```python
from build123d import *

# Parameters (mm, degrees)
BASE_FLANGE1_DEPTH    = 2
EDGE_FLANGE1_DEPTH    = 12
M5_CLEARANCE_HOLE1_D  = 5.8
M3_CLEARANCE_HOLE1_D  = 3.6
SKETCH14_R            = 1.25
CUT_EXTRUDE1_DEPTH    = 41.360872141
BREAK_CORNER1_START   = -8
BREAK_CORNER1_DEPTH   = 2
BREAK_CORNER1_2_DEPTH = 2


# Read off the part's stored shape, not the designer's step: Break-Corner1
# Sheet-metal steps are written as plain solids
with BuildPart() as part:
    # Sketch1 → Base-Flange1 (new body)
    with BuildSketch(Plane(origin=(0, 0, 0), x_dir=(1, 0, 0), z_dir=(0, 1, 0))):
        with BuildLine():
            Line((0, 0), (0, 12))
            Line((0, 12), (-34, 12))
            Line((-34, 12), (-34, 0))
            Line((-34, 0), (-13, -13))
            Line((-13, -13), (-10, -13))
            Line((-10, -13), (-10, -1))
            ThreePointArc((-10, -1), (-10.5, -0.5), (-10, 0))
            Line((-10, 0), (0, 0))
        make_face()
    extrude(amount=BASE_FLANGE1_DEPTH)

    # Edge-Flange1 section (across the edge) → Edge-Flange1 (add)
    with BuildSketch(Plane(origin=(-8, 0, 1), x_dir=(-1, 0, 0), z_dir=(0, 0, 1))):
        with BuildLine():
            Line((-2, 2), (-2, 26))
            Line((-2, 26), (0, 26))
            Line((0, 26), (0, 2))
            ThreePointArc((0, 2), (0.585786438, 0.585786438), (2, 0))
            Line((2, 0), (2, -2))
            ThreePointArc((2, -2), (-0.828427125, -0.828427125), (-2, 2))
        make_face()
    extrude(amount=EDGE_FLANGE1_DEPTH)

    # M5 Clearance Hole1 (through all)
    with Locations(Plane(origin=(0, 2, 0), x_dir=(1, 0, 0), z_dir=(0, 1, 0))):
        with Locations((-29, 6), (-5, 6)):
            Hole(M5_CLEARANCE_HOLE1_D / 2)

    # M3 Clearance Hole1 (through all)
    with Locations(Plane(origin=(-6, 0, 0), x_dir=(0, 0, -1), z_dir=(1, 0, 0))):
        with Locations((-7, -21)):
            Hole(M3_CLEARANCE_HOLE1_D / 2)

    # Sketch14 → Cut-Extrude1 (cut, through all)
    with BuildSketch(Plane(origin=(-6, 0, 0), x_dir=(0, 0, -1), z_dir=(1, 0, 0))):
        with Locations(Location((-7, -5, 0), (0, 0, 90))):
            Circle(SKETCH14_R)
    extrude(amount=-CUT_EXTRUDE1_DEPTH, mode=Mode.SUBTRACT)

    # Break-Corner1 outline → Break-Corner1 (cut)
    with BuildSketch(Plane.YZ.offset(BREAK_CORNER1_START)):
        with BuildLine():
            Line((-26, 1), (-24, 1))
            ThreePointArc((-24, 1), (-25.414213562, 1.585786438), (-26, 3))
            Line((-26, 3), (-26, 1))
        make_face()
        with BuildLine():
            Line((-26, 13), (-26, 11))
            ThreePointArc((-26, 11), (-25.414213562, 12.414213562), (-24, 13))
            Line((-24, 13), (-26, 13))
        make_face()
    extrude(amount=BREAK_CORNER1_DEPTH, mode=Mode.SUBTRACT)

    # Break-Corner1 2 outline → Break-Corner1 2 (cut)
    with BuildSketch(Plane(origin=(0, 0, 0), x_dir=(1, 0, 0), z_dir=(0, 1, 0))):
        with BuildLine():
            Line((-13, -13), (-12.431049528, -13))
            ThreePointArc((-12.431049528, -13), (-12.978287782, -12.923676244), (-13.483758757, -12.700530293))
            Line((-13.483758757, -12.700530293), (-13, -13))
        make_face()
        with BuildLine():
            Line((0, 0), (0, 2))
            ThreePointArc((0, 2), (-0.585786438, 0.585786438), (-2, 0))
            Line((-2, 0), (0, 0))
        make_face()
        with BuildLine():
            Line((0, 12), (-2, 12))
            ThreePointArc((-2, 12), (-0.585786438, 11.414213562), (0, 10))
            Line((0, 10), (0, 12))
        make_face()
        with BuildLine():
            Line((-34, 12), (-34, 10))
            ThreePointArc((-34, 10), (-33.414213562, 11.414213562), (-32, 12))
            Line((-32, 12), (-34, 12))
        make_face()
        with BuildLine():
            Line((-34, 0), (-33.052709229, -0.586418096))
            ThreePointArc((-33.052709229, -0.586418096), (-33.747200398, 0.14082356), (-34, 1.114112197))
            Line((-34, 1.114112197), (-34, 0))
        make_face()
    extrude(amount=BREAK_CORNER1_2_DEPTH, mode=Mode.SUBTRACT)


solid = part.part
```
The listing builds one solid part. Answer for the finished solid, in the listing's coordinates (mm). A direction names the side the tool comes from. Give positions to 0.01 mm unless a question says otherwise; leave off trailing zeros. Write each loop counter-clockwise with the first axis right and the second up, starting at its lowest first coordinate (ties: lowest second). Pieces come first, ordered by that corner, then holes. Notation, with made-up numbers: (1.5, -24) - (35.5, -24) arc R35 ccw to (35.5, 13) - close; hole circle Ø2 at (-27, 43). An arc over 180 degrees is marked (long way). Use one line per item in the form item = value. Start each with the question number.
1) Find section B-B on x = -5. Determine the outline of the cut face in (y, z), plus the area to 3 significant figures.
2) Find section C-C on y = -5. Determine the outline of the cut face in (x, z).
3) The mould has two halves that part along Z. Classify faces 1 (the face through (-17, 1, -12)), 2 (the face through (-12.971, 0.986, 12.926)), 3 (the face through (-10.5, 1, 0.5)): pulls with the +Z half, pulls with the -Z half, needs draft (parallel to the pull), parting line crosses it, or undercut.
4) Find section A-A on z = -6. Determine the outline of the cut face in (x, y).
5) Find section D-D on z = 10.25. Determine the outline of the cut face in (x, y), plus the area to 3 significant figures.
6) Consider line 1 along Z through (x, y) = (-7, -5); line 2 along Z through (x, y) = (-5, 0.8); line 3 along X through (y, z) = (0.75, -8.25). Determine where each line is inside the solid, lowest interval first. Write a range as from..to.
7) Flat-ended cylindrical pins translate along their axes: pin 1 Ø2 at (x, z) = (-25, -5.5) entering from -Y; pin 2 Ø9.5 at (y, z) = (-10.5, 8) entering from +X; pin 3 Ø4.5 at (x, y) = (-8, -10) entering from -Z. Find the tip coordinate at first contact, or state that the pin passes through.
8) A tool of negligible diameter and unlimited length cuts with its end or side. For faces 4 (the face through (-6, 1, 0)), 5 (the face through (-8, -14, 7)), 6 (the face through (-7.203, 0.859, 6.916)), from which of +Z, -Z, +X, -X, +Y, -Y can it reach the whole face along a straight path? Write none if from no direction.
Geometry results:
q1.outline = (0, -12) - (2, -12) - (2, -8.9) - (0, -8.9) - close; (0, -3.1) - (2, -3.1) - (2, 0) - (0, 0) - close
q1.area = 12.4 mm2
q2.outline = (-8, 1) - (-6, 1) - (-6, 5.75) - (-8, 5.75) - close; (-8, 8.25) - (-6, 8.25) - (-6, 13) - (-8, 13) - close
q3.face_1 = pulls with the -Z half
q3.face_2 = pulls with the +Z half
q3.face_3 = undercut
q4.outline = (-34, 0) - (-31.9, 0) - (-31.9, 2) - (-34, 2) - close; (-26.1, 0) - (-7.9, 0) - (-7.9, 2) - (-26.1, 2) - close; (-2.1, 0) - (0, 0) - (0, 2) - (-2.1, 2) - close
q5.outline = (-17.44, 0) - (-10, 0) arc R2 cw to (-8, -2) - (-8, -26) - (-6, -26) - (-6, -2) arc R4 ccw to (-10, 2) - (-17.44, 2) - close
q5.area = 72.3 mm2
q6.line_1 = 1..5.75, 8.25..13
q6.line_2 = -12..-8.9, -3.1..0
q6.line_3 = -34..-30.83, -27.17..-6.83, -3.17..0
q7.pin_1 = 0
q7.pin_2 = -6
q7.pin_3 = 1
q8.face_4 = +X, +Y, -Y
q8.face_5 = +Z, -Z, -X, -Y
q8.face_6 = +Z, +X, +Y
